```python
from build123d import *

# Parameters (mm, degrees)
F0_R     = 12.7
F1_DEPTH = 457.2


with BuildPart() as f1:
    # F0 (on Right) → F1 (new body)
    with BuildSketch(Plane.YZ):
        Circle(F0_R)
        Polygon((-3.662843, 6.351922), (3.669504, 6.348076), (7.332347, -0.003845), (3.662843, -6.351922), (-3.669504, -6.348076), (-7.332347, 0.003845), align=None, mode=Mode.SUBTRACT)
    extrude(amount=F1_DEPTH)


solid = f1.part
```
For this review, take the finished solid that the model builds, in its own axes (mm). Coordinates: 2 decimals unless noted, no trailing zeros. Loops run counter-clockwise (first coordinate to the right, second up) from the corner with the lowest first, then second, coordinate; pieces in that order, holes last. Notation, with made-up numbers: (-1, -10.75) -> (20, -10.75) arc R25 cw to (20, 3.25) -> close; hole circle Ø4 at (-17.75, -29.75). An arc over 180 degrees is marked (long way). Return JSON: item names as keys, results as strings. Group by question number.
(1) Consider section A-A, the plane x = 266. Give the boundary of the cut face in (y, z), plus the area to 3 significant figures.
(2) For pin 1 Ø12 at (y, z) = (0, -1.5) entering from +X; pin 2 Ø10 at (x, z) = (100.5, -6) entering from -Y; pin 3 Ø2 at (x, z) = (95.5, -9) entering from +Y; pin 4 Ø4 at (x, y) = (211.5, 8.5) entering from -Z, all flat-tipped, find the tip position at first contact; note any pin that passes through.
(3) To check wall thickness, follow L1, parallel to Y at x = 398.5, z = 5; L2, parallel to Y at x = 88, z = -4; L3, parallel to Z at x = 329.5, y = 2.5. State the ranges of each line that lie inside material, in increasing order.
Results below:
{
 "1": {"outline": "circle Ø25.4 at (0, 0); hole (-7.33, 0) -> (-3.67, -6.35) -> (3.66, -6.35) -> (7.33, 0) -> (3.67, 6.35) -> (-3.66, 6.35) -> close", "area": "367 mm2"},
 "2": {"pin 1": "stops at x = 457.2", "pin 2": "stops at y = -12.66", "pin 3": "stops at y = 9.86", "pin 4": "stops at z = -10.91"},
 "3": {"L1": "y = -11.67 to -4.44, 4.45 to 11.67", "L2": "y = -12.05 to -5.02, 5.02 to 12.05", "L3": "z = -12.45 to -6.35, 6.35 to 12.45"}
}
